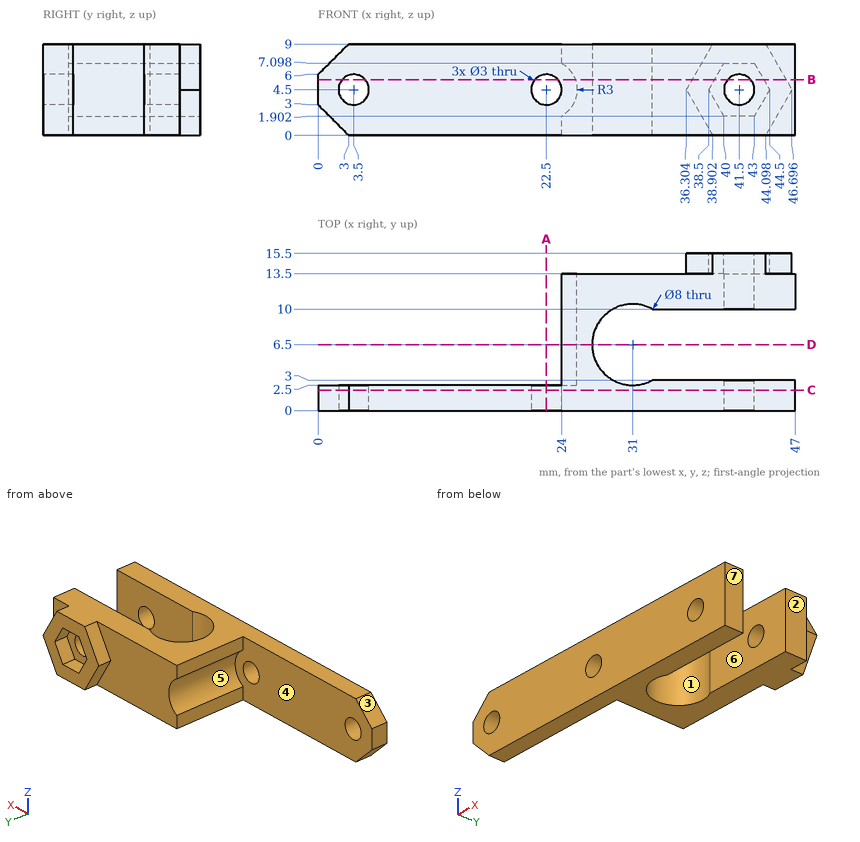
Could you check a few things on this drawing? It's one solid part, dimensions in mm from its lowest x, y, z. A direction names the side the tool comes from. Coordinates: 2 decimals unless noted, no trailing zeros. Order: outer loops, then holes, each group sorted by start corner. A loop starts at its lowest first (then second) coordinate and runs counter-clockwise, first axis right, second up. Notation, with made-up numbers: (59, 19.5) -> (80, 19.5) arc R20 ccw to (80, 47.5) -> close; hole circle Ø3 at (56, 81.25). An arc over 180 degrees is marked (long way). Answer in a Markdown table with one row per item.
(1) I want a section at B-B on z = 5.5. Count the separate pieces of the cut face and the enclosed holes in it.
Answer key:
| item | result |
|---|---|
| separate pieces | 5 |
| enclosed holes | 0 |
(2) I want a section at C-C on y = 2. List the corners of the cut face in (x, z) for me, then the cut area to 3 significant figures.
Answer key:
| item | result |
|---|---|
| outline | (0, 3) -> (3, 0) -> (47, 0) -> (47, 9) -> (3, 9) -> (0, 6) -> close; hole circle Ø3 at (3.5, 4.5); hole circle Ø3 at (22.5, 4.5); hole circle Ø3 at (41.5, 4.5) |
| area | 393 mm^2 |
(3) On a 3-axis mill with a long thin cutter (end or side, diameter ignored), from which of +Z, -Z, +X, -X, +Y, -Y can I reach the whole of each face in a straight line? I mean the marked faces 5, 6 and 7. Say none if no direction works.
Answer key:
| item | result |
|---|---|
| face 5 | -X, +Y |
| face 6 | +Z, -Z, +X |
| face 7 | +Z, -Z, +X, +Y, -Y |
(4) Will these pins go through, and if not, where does the flat tip stop? pin 1 Ø2.5 at (x, z) = (41.5, 4.5) entering from -Y; pin 2 Ø1 at (y, z) = (10, 8.5) entering from -X; pin 3 Ø2 at (y, z) = (14, 6) entering from -X (1 decimal).
Answer key:
| item | result |
|---|---|
| pin 1 | through |
| pin 2 | x = 24 |
| pin 3 | x = 24.3 |
(5) Please list where these lines run through material, in increasing order: probe 1 along Y at (x, z) = (36, 3); probe 2 along Z at (x, y) = (41.5, 0.85); probe 3 along Y at (x, z) = (25, 8.5).
Answer key:
| item | result |
|---|---|
| probe 1 | 0 to 3, 10 to 13.5 |
| probe 2 | 0 to 3, 6 to 9 |
| probe 3 | 0 to 13.5 |
(6) Thinking about a two-plate mould opening in X: for the marked faces 1, 2, 3 and 4, which applies, +X half, -X half, draft (parallel to the pull), parting line (faces both ways), or undercut?
Answer key:
| item | result |
|---|---|
| face 1 | undercut |
| face 2 | +X half |
| face 3 | -X half |
| face 4 | draft |
(7) I want a section at A-A on x = 22.5. List the corners of the cut face in (y, z) for me.
Answer key:
| item | result |
|---|---|
| outline | (0, 0) -> (2.5, 0) -> (2.5, 3) -> (0, 3) -> close; (0, 6) -> (2.5, 6) -> (2.5, 9) -> (0, 9) -> close |
(8) I want a section at D-D on y = 6.5. List the corners of the cut face in (x, z) for me.
Answer key:
| item | result |
|---|---|
| outline | (24, 0) -> (27, 0) -> (27, 9) -> (24, 9) -> (24, 7.1) arc R3 cw to (24, 1.9) -> close |
